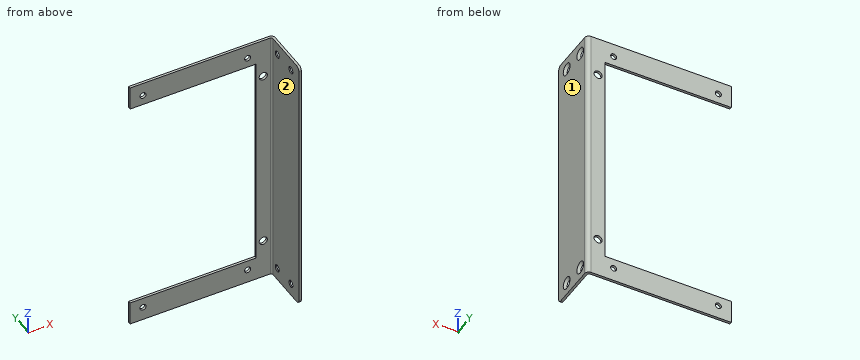
```python
from build123d import *

# Parameters (mm, degrees)
SKETCH1_W                                            = 71.22
SKETCH1_H                                            = 132.04
BASE_FLANGE1_DEPTH                                   = 1.2192
EDGE_FLANGE1_STRIP_W                                 = 6.3968
EDGE_FLANGE1_STRIP_H                                 = 1.2192
EDGE_FLANGE1_STRIP_CUT_DEPTH                         = 132.04
EDGE_FLANGE1_DEPTH                                   = 132.04
CUT_EXTRUDE2_REACH                                   = 154.088
SKETCH28_W                                           = 62.22
SKETCH28_H                                           = 108.5
CSK_FOR_M3_CROSS_COUNTERSUNK_HEAD_SCREW4_D           = 3.4
CSK_FOR_M3_CROSS_COUNTERSUNK_HEAD_SCREW4_CSINK_D     = 6
CSK_FOR_M3_CROSS_COUNTERSUNK_HEAD_SCREW4_CSINK_ANGLE = 92
F_3_0MM_DOWEL_HOLE1_D                                = 3
CUT_EXTRUDE3_REACH                                   = 154.088
F_4_0MM_DOWEL_HOLE1_D                                = 4


# Sheet-metal steps are written as plain solids
with BuildPart() as part:
    # Sketch1 → Base-Flange1 (new body)
    with BuildSketch(Plane(origin=(0, 0, 0), x_dir=(1, 0, 0), z_dir=(0, 1, 0))):
        with Locations((35.61, 66.02)):
            Rectangle(SKETCH1_W, SKETCH1_H)
    extrude(amount=-BASE_FLANGE1_DEPTH)

    # Edge-Flange1 strip (across the edge) → Edge-Flange1 strip cut (cut)
    with BuildSketch(Plane(origin=(71.22, -1.2192, -132.04), x_dir=(-1, 0, 0), z_dir=(0, 0, 1))):
        with Locations((-1.2192, -0.6096)):
            Rectangle(EDGE_FLANGE1_STRIP_W, EDGE_FLANGE1_STRIP_H)
    extrude(amount=EDGE_FLANGE1_STRIP_CUT_DEPTH, mode=Mode.SUBTRACT)

    # Edge-Flange1 section (across the edge) → Edge-Flange1 (add)
    with BuildSketch(Plane(origin=(71.22, -1.2192, -132.04), x_dir=(-1, 0, 0), z_dir=(0, 0, 1))):
        with BuildLine():
            Line((0, 0.76), (0, 23.76))
            Line((0, 23.76), (1.2192, 23.76))
            Line((1.2192, 23.76), (1.2192, 0.76))
            ThreePointArc((1.2192, 0.76), (1.441798846, 0.222598846), (1.9792, 0))
            Line((1.9792, 0), (1.9792, -1.2192))
            ThreePointArc((1.9792, -1.2192), (0.579694259, -0.639505741), (0, 0.76))
        make_face()
    extrude(amount=EDGE_FLANGE1_DEPTH)

    # Sketch28 → Cut-Extrude2 (cut, up to next)
    with BuildSketch(Plane(origin=(0, 0, 0), x_dir=(1, 0, 0), z_dir=(0, 1, 0)), mode=Mode.PRIVATE) as cut_extrude2_sk1:
        with Locations((31.11, 66.02)):
            Rectangle(SKETCH28_W, SKETCH28_H)
    cut_extrude2_tool1 = extrude(cut_extrude2_sk1.sketch, amount=-CUT_EXTRUDE2_REACH, mode=Mode.PRIVATE) & part.part
    add(cut_extrude2_tool1.solids().sort_by_distance((31.11, 0, -66.02))[0], mode=Mode.SUBTRACT)

    # CSK for M3 Cross Countersunk Head Screw4 (through all)
    with Locations(Plane(origin=(71.22, -5.9492, -6.22), x_dir=(0, 1, 0), z_dir=(1, 0, 0))):
        with Locations((0, 0), (-12, 0), (0, -119.6), (-12, -119.6)):
            CounterSinkHole(CSK_FOR_M3_CROSS_COUNTERSUNK_HEAD_SCREW4_D / 2, CSK_FOR_M3_CROSS_COUNTERSUNK_HEAD_SCREW4_CSINK_D / 2, counter_sink_angle=CSK_FOR_M3_CROSS_COUNTERSUNK_HEAD_SCREW4_CSINK_ANGLE)

    # Ø3.0mm Dowel Hole1 (through all)
    with Locations(Plane(origin=(6.41, 0, -125.27), x_dir=(0, 0, 1), z_dir=(0, 1, 0))):
        with Locations((0, 0), (0, 51.62), (118.5, 51.62), (118.5, 0)):
            Hole(F_3_0MM_DOWEL_HOLE1_D / 2)

    # Sketch35 → Cut-Extrude3 (cut, up to next)
    with BuildSketch(Plane(origin=(71.22, 0, 0), x_dir=(0, 0, -1), z_dir=(1, 0, 0)), mode=Mode.PRIVATE) as cut_extrude3_sk1:
        with BuildLine():
            Line((0, -24.9792), (1.98, -24.9792))
            ThreePointArc((1.98, -24.9792), (0.579928573, -24.399271427), (0, -22.9992))
            Line((0, -22.9992), (0, -24.9792))
        make_face()
    cut_extrude3_tool1 = extrude(cut_extrude3_sk1.sketch, amount=-CUT_EXTRUDE3_REACH, mode=Mode.PRIVATE) & part.part
    # Sketch35 → Cut-Extrude3 (cut, up to next)
    with BuildSketch(Plane(origin=(71.22, 0, 0), x_dir=(0, 0, -1), z_dir=(1, 0, 0)), mode=Mode.PRIVATE) as cut_extrude3_sk2:
        with BuildLine():
            Line((132.04, -24.9792), (130.06, -24.9792))
            ThreePointArc((130.06, -24.9792), (131.460071427, -24.399271427), (132.04, -22.9992))
            Line((132.04, -22.9992), (132.04, -24.9792))
        make_face()
    cut_extrude3_tool2 = extrude(cut_extrude3_sk2.sketch, amount=-CUT_EXTRUDE3_REACH, mode=Mode.PRIVATE) & part.part
    add(cut_extrude3_tool1.solids().sort_by_distance((71.22, -24.536931, -0.442269))[0], mode=Mode.SUBTRACT)
    add(cut_extrude3_tool2.solids().sort_by_distance((71.22, -24.536931, -131.597731))[0], mode=Mode.SUBTRACT)

    # Ø4.0mm Dowel Hole1 (through all)
    with Locations(Plane(origin=(0, 0, 0), x_dir=(1, 0, 0), z_dir=(0, 1, 0))):
        with Locations((65.72, 112.04), (65.72, 20)):
            Hole(F_4_0MM_DOWEL_HOLE1_D / 2)


solid = part.part
```
The listing builds one solid part. Answer for the finished solid, in the listing's coordinates (mm). Face numbers are marked on the shaded views. A direction names the side the tool comes from. Coordinates: 2 decimals unless noted, no trailing zeros. Write each loop counter-clockwise with the first axis right and the second up, starting at its lowest first coordinate (ties: lowest second). Pieces come first, ordered by that corner, then holes. Notation, with made-up numbers: (-39, 19) -> (6, 19) arc R24 ccw to (6, 42) -> close; hole circle Ø10 at (7.25, 55.5). An arc over 180 degrees is marked (long way). Write each question's results on one line, items separated by ' | '. Start each with the question number.
1) Straight lines are drawn through the part: probe 1 along Z at (x, y) = (65.72, -0.9); probe 2 along X at (y, z) = (-0.35, -6.77); probe 3 along Y at (x, z) = (63, -6). For each, find the intervals that lie inside material, in ascending order.
2) A cutting plane is placed at D-D (z = -41.5). Determine the outline of the cut face in (x, y), then the cut area to 3 significant figures.
3) A tool of negligible diameter and unlimited length cuts with its end or side. For the marked faces 1 and 2, from which of +Z, -Z, +X, -X, +Y, -Y can it reach the whole face along a straight path? Write none if from no direction.
4) Flat-ended cylindrical pins translate along their axes: pin 1 Ø5 at (y, z) = (-14, -89) entering from -X; pin 2 Ø6.5 at (x, z) = (65.72, -112.04) entering from -Y; pin 3 Ø1 at (y, z) = (-0.5, -60.5) entering from -X. Find the tip coordinate at first contact, or state that the pin passes through.
5) A cutting plane is placed at A-A (z = -112.04). Determine the outline of the cut face in (x, y).
6) A cutting plane is placed at B-B (x = 65.72). Determine the outline of the cut face in (y, z).
7) A cutting plane is placed at C-C (x = 28.5). Determine the outline of the cut face in (y, z).
Values follow:
1) probe 1: -132.04 to -114.04, -110.04 to -22, -18 to 0 | probe 2: 0 to 4.91, 7.91 to 56.53, 59.53 to 70.36 | probe 3: -1.22 to 0
2) outline: (62.22, -1.22) -> (69.24, -1.22) arc R0.76 cw to (70, -1.98) -> (70, -24.98) -> (71.22, -24.98) -> (71.22, -1.98) arc R1.98 ccw to (69.24, 0) -> (62.22, 0) -> close | area: 39.2 mm²
3) face 1: +Z, -Z, +X, +Y, -Y | face 2: +Z, -Z, -X, -Y
4) pin 1: x = 70 | pin 2: y = -1.22 | pin 3: x = 62.22
5) outline: (62.22, -1.22) -> (63.72, -1.22) -> (63.72, 0) -> (62.22, 0) -> close; (67.72, -1.22) -> (69.24, -1.22) arc R0.76 cw to (70, -1.98) -> (70, -24.98) -> (71.22, -24.98) -> (71.22, -1.98) arc R1.98 ccw to (69.24, 0) -> (67.72, 0) -> close
6) outline: (-1.22, -132.04) -> (0, -132.04) -> (0, -114.04) -> (-1.22, -114.04) -> close; (-1.22, -110.04) -> (0, -110.04) -> (0, -22) -> (-1.22, -22) -> close; (-1.22, -18) -> (0, -18) -> (0, 0) -> (-1.22, 0) -> close
7) outline: (-1.22, -132.04) -> (0, -132.04) -> (0, -120.27) -> (-1.22, -120.27) -> close; (-1.22, -11.77) -> (0, -11.77) -> (0, 0) -> (-1.22, 0) -> close
